Input: part model. Units: mm. Frame: model coordinates. Give positions to 0.01 mm unless a question says otherwise; leave off trailing zeros. Order: outer loops, then holes, each group sorted by start corner. A loop starts at its lowest first (then second) coordinate and runs counter-clockwise, first axis right, second up. Notation, with made-up numbers: M -22,73.5 L -7,73.5 A5 ccw -7,82.5 Z; hole C 27,61.5 d3. An arc over 180 degrees is marked long. Use a Markdown table: item, result.
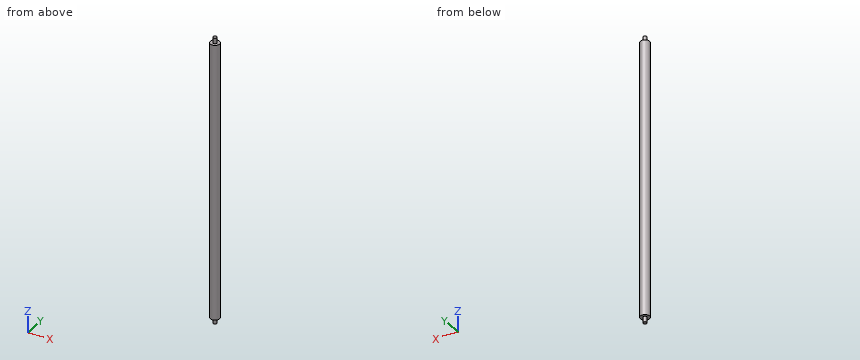
Autodesk Inventor part; units mm, degrees
ref_plane "YZ Plane" through (0, 0, 0) normal (1, 0, 0) x (0, 1, 0)
ref_plane "XZ Plane" through (0, 0, 0) normal (0, 1, 0) x (-1, 0, 0)
ref_plane "XY Plane" through (0, 0, 0) normal (0, 0, 1) x (1, 0, 0)
sketch "Sketch1" plane through (0, 0, 0) normal (0, 0, 1) x (1, 0, 0)
  circle A0 centre (0, 0) radius 2.5
  dimension "d0" = 5
extrude "Extrusion1" add sketch "Sketch1" along normal blind 150
sketch "Sketch2" plane through (0, 0, 150) normal (0, 0, 1) x (1, 0, 0)
  circle A0 centre (0, 0) radius 2.5
  circle A1 centre (0, 0) radius 1
  dimension "d3" = 2
extrude "Extrusion2" add sketch "Sketch2" along normal blind 3 contours A1
sketch "Sketch3" plane through (0, 0, 0) normal (0, 0, -1) x (-1, 0, 0)
  circle A0 centre (0, 0) radius 1
  dimension "d6" = 2
extrude "Extrusion3" add sketch "Sketch3" along normal blind 3
properties part number "Bone-15cm"
1) Material intervals for line 1 (Z direction, x = 2.2, y = 1.05); line 2 (Y direction, x = 0.25, z = 144.5); line 3 (X direction, y = -0.3, z = 67), sorted ascending. Write a range as from..to.
Response values:
| item | result |
|---|---|
| line 1 | z = 0..150 |
| line 2 | y = -2.49..2.49 |
| line 3 | x = -2.48..2.48 |
2) First-contact query: pin 1 Ø1.5 at (x, z) = (2, 53.5) entering from -Y; pin 2 Ø1.5 at (y, z) = (-1.5, 88.5) entering from +X. Flat tips, straight axial feed; report the tip coordinate or a pass-through.
Response values:
| item | result |
|---|---|
| pin 1 | stops at y = -2.17 |
| pin 2 | stops at x = 2.38 |
3) Cut plane A-A on y = 0. Return loops of the section in (x, z).
Response values:
| item | result |
|---|---|
| outline | M -2.5,0 L -1,0 L -1,-3 L 1,-3 L 1,0 L 2.5,0 L 2.5,150 L 1,150 L 1,153 L -1,153 L -1,150 L -2.5,150 Z |
4) Cut plane C-C on z = 72.5. Return loops of the section in (x, y).
Response values:
| item | result |
|---|---|
| outline | C 0,0 d5 |
